Check sheet for the modelled part. Datum: model origin and axes. Units: mm. A direction names the side the tool comes from. Round coordinates to 2 decimals unless told otherwise and drop trailing zeros. Write each loop counter-clockwise with the first axis right and the second up, starting at its lowest first coordinate (ties: lowest second). Pieces come first, ordered by that corner, then holes. Notation, with made-up numbers: (67.25, 49.25) - (106.25, 49.25) arc R22 cw to (106.25, 69.25) - close; hole circle Ø3 at (30, 17.5). An arc over 180 degrees is marked (long way). Use one line per item in the form item = value. Start each with the question number.
1) Section check D-D (x = -10). Record the boundary of the cut face in (y, z).
2) Scan lines: probe 1 along Y at (x, z) = (47, 30); probe 2 along X at (y, z) = (15.5, 4); probe 3 along Y at (x, z) = (-43.5, 18). Record each from-to range of solid material in increasing order.
3) Section check A-A (x = 51). Record the boundary of the cut face in (y, z).
4) Draft check along Y on faces 5 (the face through (-56.133, -26.034, 35.21)), 6 (the face through (61.58, -31.39, 34.51)), 7 (the face through (56.034, 26.133, 35.21)). Enter one of: +Y half, -Y half, draft (parallel to the pull), parting line (faces both ways), or undercut.
5) Section check B-B (z = 63). Record the boundary of the cut face in (x, y), then the cut area to 3 significant figures.
6) Set-up check for faces 1 (the face through (56.034, -26.133, 35.21)), 2 (the face through (-43.25, 21.05, 18.48)), 3 (the face through (55, 0, 54)), 4 (the face through (51, -23, 17)): record each of +Z, -Z, +X, -X, +Y, -Y from which the full face is reachable in a straight line by a thin tool's end or side.
7) Section check C-C (y = -12.5). Record the boundary of the cut face in (x, z).
8) Gauge pin test, flat ends, axial feed: P1, Ø3.5, axis at x = -55.5, z = 19, coming from the -Y side; P2, Ø2.5, axis at x = 56, z = 19, coming from the -Y side; P3, Ø6, axis at x = 46.05, y = 20.94, coming from the -Z side. Record the tip position at first contact, or that the pin passes through.
from build123d import *

# Parameters (mm, degrees)
EXTRUDE_1_DEPTH     = 70
CUT_EXTRUDE_1_DEPTH = 70
EXTRUDE_2_DEPTH     = 20
CUT_EXTRUDE_2_DEPTH = 15
EXTRUDE_3_DEPTH     = 50
SKETCH_5_R          = 1.45
CUT_EXTRUDE_3_DEPTH = 15
FILLET_1_R          = 2
EXTRUDE_4_DEPTH     = 3
SKETCH_7_R          = 2.5
CUT_EXTRUDE_4_DEPTH = 4


with BuildPart() as part:
    # Sketch 1 → Extrude 1 (new body)
    with BuildSketch(Plane.XY):
        with BuildLine():
            Line((-53, 35), (53, 35))
            ThreePointArc((53, 35), (61.485281374, 31.485281374), (65, 23))
            Line((65, 23), (65, -23))
            ThreePointArc((65, -23), (61.485281374, -31.485281374), (53, -35))
            Line((53, -35), (-53, -35))
            ThreePointArc((-53, -35), (-61.485281374, -31.485281374), (-65, -23))
            Line((-65, -23), (-65, 23))
            ThreePointArc((-65, 23), (-61.485281374, 31.485281374), (-53, 35))
        make_face()
    extrude(amount=EXTRUDE_1_DEPTH)

    # Sketch 2 → Cut-Extrude 1 (cut)
    with BuildSketch(Plane.XY.offset(70)):
        with BuildLine():
            Line((-53, -30), (53, -30))
            ThreePointArc((53, -30), (57.949747468, -27.949747468), (60, -23))
            Line((60, -23), (60, 23))
            ThreePointArc((60, 23), (57.949747468, 27.949747468), (53, 30))
            Line((53, 30), (-53, 30))
            ThreePointArc((-53, 30), (-57.949747468, 27.949747468), (-60, 23))
            Line((-60, 23), (-60, -23))
            ThreePointArc((-60, -23), (-57.949747468, -27.949747468), (-53, -30))
        make_face()
    extrude(amount=-CUT_EXTRUDE_1_DEPTH, mode=Mode.SUBTRACT)

    # Sketch 3 → Extrude 2 (add)
    with BuildSketch(Plane.XY.offset(70)):
        with BuildLine():
            Line((-53, -30), (53, -30))
            ThreePointArc((53, -30), (57.949747468, -27.949747468), (60, -23))
            Line((60, -23), (60, 23))
            ThreePointArc((60, 23), (57.949747468, 27.949747468), (53, 30))
            Line((53, 30), (-53, 30))
            ThreePointArc((-53, 30), (-57.949747468, 27.949747468), (-60, 23))
            Line((-60, 23), (-60, -23))
            ThreePointArc((-60, -23), (-57.949747468, -27.949747468), (-53, -30))
        make_face()
        with BuildLine():
            Line((-53, -25), (53, -25))
            ThreePointArc((53, -25), (54.414213562, -24.414213562), (55, -23))
            Line((55, -23), (55, 23))
            ThreePointArc((55, 23), (54.414213562, 24.414213562), (53, 25))
            Line((53, 25), (-53, 25))
            ThreePointArc((-53, 25), (-54.414213562, 24.414213562), (-55, 23))
            Line((-55, 23), (-55, -23))
            ThreePointArc((-55, -23), (-54.414213562, -24.414213562), (-53, -25))
        make_face(mode=Mode.SUBTRACT)
    extrude(amount=-EXTRUDE_2_DEPTH)

    # Sketch 3_2 → Cut-Extrude 2 (cut)
    with BuildSketch(Plane.XY.offset(70)):
        with BuildLine():
            Line((-53, -30), (53, -30))
            ThreePointArc((53, -30), (57.949747468, -27.949747468), (60, -23))
            Line((60, -23), (60, 23))
            ThreePointArc((60, 23), (57.949747468, 27.949747468), (53, 30))
            Line((53, 30), (-53, 30))
            ThreePointArc((-53, 30), (-57.949747468, 27.949747468), (-60, 23))
            Line((-60, 23), (-60, -23))
            ThreePointArc((-60, -23), (-57.949747468, -27.949747468), (-53, -30))
        make_face()
        with BuildLine():
            Line((-53, -25), (53, -25))
            ThreePointArc((53, -25), (54.414213562, -24.414213562), (55, -23))
            Line((55, -23), (55, 23))
            ThreePointArc((55, 23), (54.414213562, 24.414213562), (53, 25))
            Line((53, 25), (-53, 25))
            ThreePointArc((-53, 25), (-54.414213562, 24.414213562), (-55, 23))
            Line((-55, 23), (-55, -23))
            ThreePointArc((-55, -23), (-54.414213562, -24.414213562), (-53, -25))
        make_face(mode=Mode.SUBTRACT)
    extrude(amount=-CUT_EXTRUDE_2_DEPTH, mode=Mode.SUBTRACT)

    # Sketch 4 → Extrude 3 (add)
    with BuildSketch(Plane(origin=(0, 0, 50), x_dir=(-1, 0, 0), z_dir=(0, 0, -1))):
        with BuildLine():
            ThreePointArc((-53, 30), (-56.083662278, 26.083662278), (-60, 23))
            ThreePointArc((-60, 23), (-57.949747468, 27.949747468), (-53, 30))
        make_face()
        with BuildLine():
            ThreePointArc((53, 30), (56.083662278, 26.083662278), (60, 23))
            ThreePointArc((60, 23), (57.949747468, 27.949747468), (53, 30))
        make_face()
        with BuildLine():
            ThreePointArc((53, -30), (57.949747468, -27.949747468), (60, -23))
            ThreePointArc((60, -23), (56.083662278, -26.083662278), (53, -30))
        make_face()
        with BuildLine():
            ThreePointArc((-53, -30), (-56.083662278, -26.083662278), (-60, -23))
            ThreePointArc((-60, -23), (-57.949747468, -27.949747468), (-53, -30))
        make_face()
    extrude(amount=EXTRUDE_3_DEPTH)

    # Sketch 5 → Cut-Extrude 3 (cut)
    with BuildSketch(Plane(origin=(0, 0, 0), x_dir=(-1, 0, 0), z_dir=(0, 0, -1))):
        with Locations((-58.865243762, 28.354943792)):
            Circle(SKETCH_5_R)
        with Locations(Location((58.865243762, 28.354943792, 0), (0, 0, 180))):
            Circle(SKETCH_5_R)
        with Locations((58.865243762, -28.354943792)):
            Circle(SKETCH_5_R)
        with Locations(Location((-58.865243762, -28.354943792, 0), (0, 0, 180))):
            Circle(SKETCH_5_R)
    extrude(amount=-CUT_EXTRUDE_3_DEPTH, mode=Mode.SUBTRACT)

    # Fillet 1
    fillet_1_edges = [part.edges().sort_by_distance(p)[0] for p in [
        (0, -25, 50),
        (54.414213562, -24.414213562, 50),
        (55, 0, 50),
        (54.414213562, 24.414213562, 50),
        (0, 25, 50),
        (-54.414213562, 24.414213562, 50),
        (-55, 0, 50),
        (-54.414213562, -24.414213562, 50),
    ]]
    fillet(fillet_1_edges, radius=FILLET_1_R)

    # Sketch 6 → Extrude 4 (add)
    with BuildSketch(Plane(origin=(0, 0, 20), x_dir=(-1, 0, 0), z_dir=(0, 0, -1))):
        with BuildLine():
            Line((61.485281374, 31.485281374), (41.485281374, 31.485281374))
            Line((41.485281374, 31.485281374), (41.485281374, 20.485281374))
            ThreePointArc((41.485281374, 20.485281374), (42.949747468, 16.949747468), (46.485281374, 15.485281374))
            Line((46.485281374, 15.485281374), (61.485281374, 15.485281374))
            Line((61.485281374, 15.485281374), (61.485281374, 31.485281374))
        make_face()
        with BuildLine():
            Line((-61.485281374, 15.485281374), (-46.485281374, 15.485281374))
            ThreePointArc((-46.485281374, 15.485281374), (-42.949747468, 16.949747468), (-41.485281374, 20.485281374))
            Line((-41.485281374, 20.485281374), (-41.485281374, 31.485281374))
            Line((-41.485281374, 31.485281374), (-61.485281374, 31.485281374))
            Line((-61.485281374, 31.485281374), (-61.485281374, 15.485281374))
        make_face()
        with BuildLine():
            Line((-61.485281374, -31.485281374), (-61.485281374, -15.485281374))
            Line((-61.485281374, -15.485281374), (-46.485281374, -15.485281374))
            ThreePointArc((-46.485281374, -15.485281374), (-42.949747468, -16.949747468), (-41.485281374, -20.485281374))
            Line((-41.485281374, -20.485281374), (-41.485281374, -31.485281374))
            Line((-41.485281374, -31.485281374), (-61.485281374, -31.485281374))
        make_face()
        with BuildLine():
            Line((61.485281374, -15.485281374), (46.485281374, -15.485281374))
            ThreePointArc((46.485281374, -15.485281374), (42.949747468, -16.949747468), (41.485281374, -20.485281374))
            Line((41.485281374, -20.485281374), (41.485281374, -31.485281374))
            Line((41.485281374, -31.485281374), (61.485281374, -31.485281374))
            Line((61.485281374, -31.485281374), (61.485281374, -15.485281374))
        make_face()
    extrude(amount=EXTRUDE_4_DEPTH)

    # Sketch 7 → Cut-Extrude 4 (cut)
    with BuildSketch(Plane(origin=(0, 0, 17), x_dir=(-1, 0, 0), z_dir=(0, 0, -1))):
        with Locations((-46.054090748, 20.935782702)):
            Circle(SKETCH_7_R)
        with Locations((45.745909252, 20.935782702)):
            Circle(SKETCH_7_R)
        with Locations((45.745909252, -20.864217298)):
            Circle(SKETCH_7_R)
        with Locations((-46.054090748, -20.864217298)):
            Circle(SKETCH_7_R)
    extrude(amount=-CUT_EXTRUDE_4_DEPTH, mode=Mode.SUBTRACT)


solid = part.part
Results are:
q1.outline = (-35, 0) - (-30, 0) - (-30, 50) - (-27, 50) arc R2 ccw to (-25, 52) - (-25, 55) - (-30, 55) - (-30, 70) - (-35, 70) - close; (25, 52) arc R2 ccw to (27, 50) - (30, 50) - (30, 0) - (35, 0) - (35, 70) - (30, 70) - (30, 55) - (25, 55) - close
q2.probe_1 = -35 to -30, 30 to 35
q2.probe_2 = -65 to -60, 60 to 65
q2.probe_3 = -35 to -21.96, -19.77 to -16.47, 16.47 to 19.84, 22.03 to 35
q3.outline = (-35, 0) - (-30, 0) - (-30, 17) - (-15.49, 17) - (-15.49, 20) - (-30, 20) - (-30, 50) - (-27, 50) arc R2 ccw to (-25, 52) - (-25, 55) - (-30, 55) - (-30, 70) - (-35, 70) - close; (15.49, 17) - (30, 17) - (30, 0) - (35, 0) - (35, 70) - (30, 70) - (30, 55) - (25, 55) - (25, 52) arc R2 ccw to (27, 50) - (30, 50) - (30, 20) - (15.49, 20) - close
q4.face_5 = undercut
q4.face_6 = -Y half
q4.face_7 = undercut
q5.outline = (-65, -23) arc R12 ccw to (-53, -35) - (53, -35) arc R12 ccw to (65, -23) - (65, 23) arc R12 ccw to (53, 35) - (-53, 35) arc R12 ccw to (-65, 23) - close; hole (-60, -23) arc R7 ccw to (-53, -30) - (53, -30) arc R7 ccw to (60, -23) - (60, 23) arc R7 ccw to (53, 30) - (-53, 30) arc R7 ccw to (-60, 23) - close
q5.area = 1,820 mm²
q6.face_1 = none
q6.face_2 = +Z, -Z
q6.face_3 = +Z
q6.face_4 = -Z
q7.outline = (-65, 0) - (-60, 0) - (-60, 50) - (-57, 50) arc R2 ccw to (-55, 52) - (-55, 55) - (-60, 55) - (-60, 70) - (-65, 70) - close; (55, 52) arc R2 ccw to (57, 50) - (60, 50) - (60, 0) - (65, 0) - (65, 70) - (60, 70) - (60, 55) - (55, 55) - close
q8.P1 = -34.98
q8.P2 = -34.87
q8.P3 = 17
